Drawing for the job (mm, zero at the part's lowest x, y, z). A direction names the side the tool comes from. Give positions to 0.01 mm unless a question says otherwise; leave off trailing zeros. Order: outer loops, then holes, each group sorted by start corner. A loop starts at its lowest first (then second) coordinate and runs counter-clockwise, first axis right, second up. Notation, with made-up numbers: (15.5, 81) -> (38.5, 81) arc R26 cw to (38.5, 112) -> close; hole circle Ø3 at (70.25, 63). An arc over 180 degrees is marked (long way). One line per item, written item: value. Start each with the question number.
(1) Saw through at B-B on x = 32. Give the cut face in (y, z).
(2) Two-plate mould, pull along X, no slides. Class the marked faces 1, 2 and 3: +X half, -X half, draft (parallel to the pull), parting line (faces both ways), or undercut.
(3) Which spindle directions (+Z, -Z, +X, -X, +Y, -Y) get a long thin tool onto all of the face, cutting with end or side? Do the marked faces 4, 5 and 6. Say none if no direction does.
(4) Pin check, flat tips, straight feed: pin 1 (4 mm diameter, centred on x = 26.5, z = 10, fed in from +Y); pin 2 (5 mm diameter, centred on y = 37.5, z = 16.5, fed in from -X); pin 3 (3 mm diameter, centred on x = 32, y = 48, fed in from -Z). Stop position of each tip, or through.
(5) Probe line 1 (Z direction, x = 14, y = 6); line 2 (X direction, y = 7.5, z = 19.5) (1 decimal); line 3 (X direction, y = 31.5, z = 28). List the from-to ranges inside material, lowest first.
(6) Saw through at D-D on z = 6. Give the cut face in (x, y).
(7) Saw through at C-C on z = 25. Give the cut face in (x, y), plus the area to 3 significant figures.
(8) Saw through at A-A on y = 32. Give the cut face in (x, z).
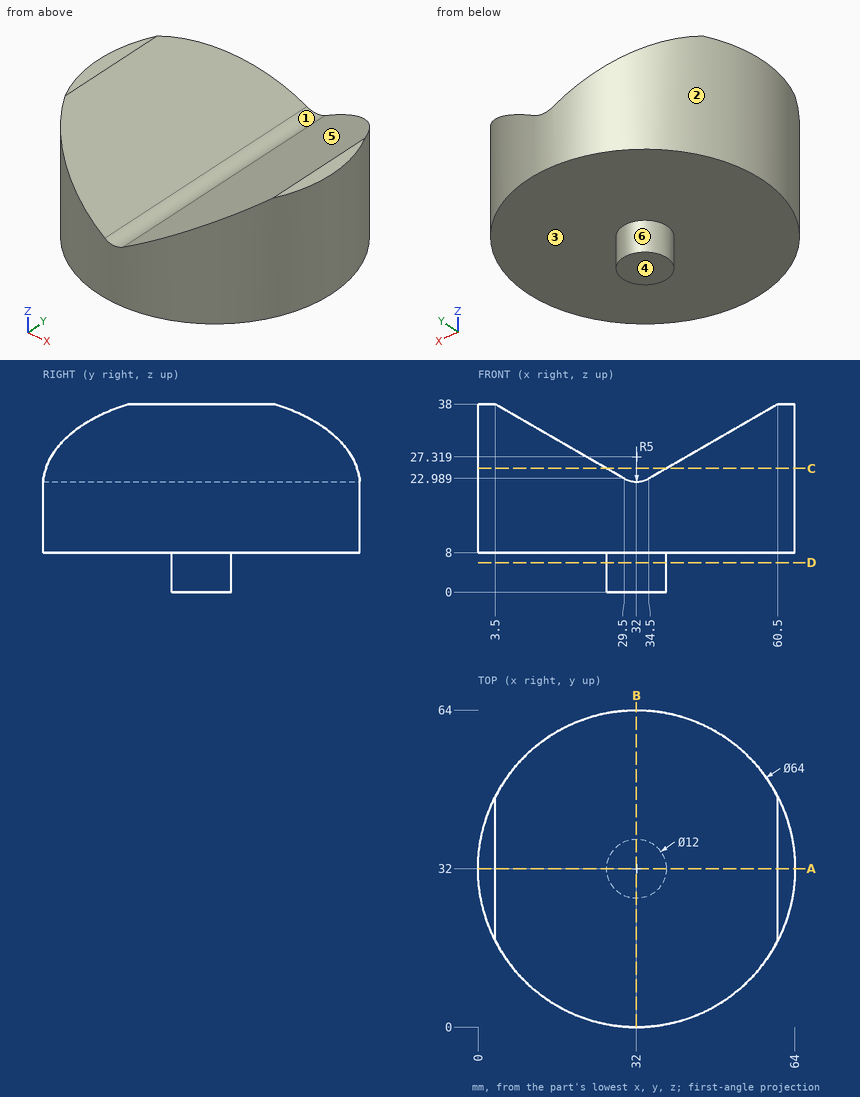
Results below:
1. outline: (0, 8) -> (26, 8) -> (26, 0) -> (38, 0) -> (38, 8) -> (64, 8) -> (64, 22.32) -> (0, 22.32) -> close
2. face 1: undercut
2. face 2: parting line
2. face 3: draft
3. face 4: -Z, +X, -X, +Y, -Y
3. face 5: +Z, +Y, -Y
3. face 6: -Z
4. pin 1: stops at y = 63.81
4. pin 2: stops at x = 0.14
4. pin 3: stops at z = 8
5. line 1: z = 8 to 31.94
5. line 2: x = 11.4 to 52.6
5. line 3: x = 0 to 20.82, 43.18 to 64
6. outline: circle Ø12 at (32, 32)
7. outline: (26.02, 0.56) -> (26.02, 63.44) arc R32 ccw to start; (37.98, 0.56) arc R32 ccw to (37.98, 63.44) -> close
7. area: 2,460 mm²
8. outline: (0, 8) -> (26, 8) -> (26, 0) -> (38, 0) -> (38, 8) -> (64, 8) -> (64, 38) -> (60.5, 38) -> (34.5, 22.99) arc R5 cw to (29.5, 22.99) -> (3.5, 38) -> (0, 38) -> close
